from build123d import *

# Parameters (mm, degrees)
F0_W     = 15.6635074461
F0_H     = 5
F1_DEPTH = 10
F2_W     = 25.6835715845
F2_H     = 20.0516330078
F3_DEPTH = 1


with BuildPart() as f1:
    # F0 (on Front) → F1 (new body)
    with BuildSketch(Plane.XZ):
        Polygon((-29.1881171715, 35.4532431718), (-34.1881171715, 35.4532431718), (-34.1881171715, 15.4532431718), (-29.1881171715, 15.4532431718), (-29.1881171715, 20.4532431718), align=None)
        with Locations((-21.3563634484, 17.9532431718)):
            Rectangle(F0_W, F0_H)
        Polygon((-13.5246097253, 35.4532431718), (-13.5246097253, 20.4532431718), (-13.5246097253, 15.4532431718), (-8.5246097253, 15.4532431718), (-8.5246097253, 35.4532431718), align=None)
    extrude(amount=F1_DEPTH)

    # F2 (on Front) → F3 (join)
    with BuildSketch(Plane.XZ):
        with Locations((-21.3003805839, 25.4549360834)):
            Rectangle(F2_W, F2_H)
    extrude(amount=F3_DEPTH)


solid = f1.part
Can you work these out from the model? Positions are in its coordinate system, mm. A direction names the side the tool comes from. Give positions to 0.01 mm unless a question says otherwise; leave off trailing zeros. Loops run counter-clockwise (first coordinate to the right, second up) from the corner with the lowest first, then second, coordinate; pieces in that order, holes last. Notation, with made-up numbers: M -11.5,33.5 L 18.5,33.5 A7 ccw 18.5,44.5 Z; hole C 25,46.25 d5. An arc over 180 degrees is marked long. One line per item, written item: value.
1) I'm going to push flat-ended pins straight in: pin 1 (4 mm diameter, centred on x = -31.5, y = -6, fed in from +Z); pin 2 (1 mm diameter, centred on x = -28, z = 32.5, fed in from -Y); pin 3 (6 mm diameter, centred on y = -8.5, z = 31.5, fed in from +X). Where does each tip first touch, or does it pass through?
Geometry check:
pin 1: stops at z = 35.45
pin 2: stops at y = -1
pin 3: stops at x = -8.52
2) Please list where these lines run through material, in increasing order: line 1 (X direction, y = -4, z = 26); line 2 (Y direction, x = -14.5, z = 23); line 3 (Z direction, x = -10.75, y = -6.5).
Geometry check:
line 1: x = -34.19 to -29.19, -13.52 to -8.52
line 2: y = -1 to 0
line 3: z = 15.45 to 35.45
3) Imagine slicing it at B-B on y = -3. Write out the boundary of the cut face in (x, z).
Geometry check:
outline: M -34.19,15.45 L -8.52,15.45 L -8.52,35.45 L -13.52,35.45 L -13.52,20.45 L -29.19,20.45 L -29.19,35.45 L -34.19,35.45 Z
4) Imagine slicing it at A-A on z = 30.75. Write out the boundary of the cut face in (x, y).
Geometry check:
outline: M -34.19,-10 L -29.19,-10 L -29.19,-1 L -13.52,-1 L -13.52,-10 L -8.52,-10 L -8.52,-1 L -8.46,-1 L -8.46,0 L -34.19,0 Z
5) On a 3-axis mill with a long thin cutter (end or side, diameter ignored), from which of +Z, -Z, +X, -X, +Y, -Y can I reach the whole of each face in a straight line? I mean faces 1 (the face through (-8.525, -5, 25)), 2 (the face through (-29.188, -5, 28)), 3 (the face through (-34.188, -5, 26)), 4 (the face through (-11, -5, 35.453)). Say none if no direction works.
Geometry check:
face 1: +Z, -Z, +X, -Y
face 2: +Z, -Y
face 3: +Z, -Z, -X, +Y, -Y
face 4: +Z, +X, -X, -Y
